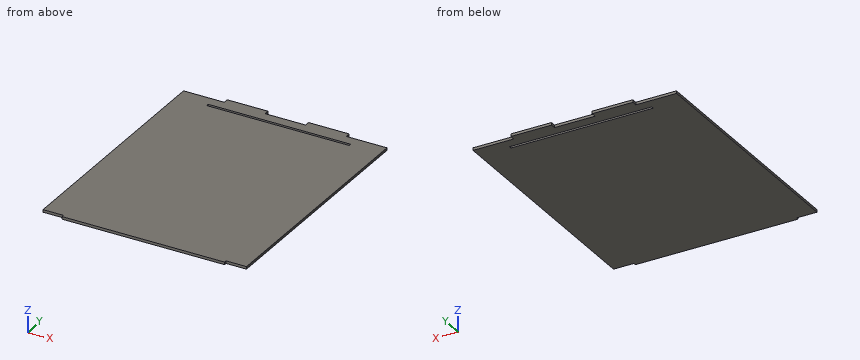
from build123d import *

# Parameters (mm, degrees)
SKETCH1_W           = 177.8
SKETCH1_H           = 3.175
BOSS_EXTRUDE1_DEPTH = 3.175


with BuildPart() as part:
    # Sketch1 → Boss-Extrude1 (new body)
    with BuildSketch(Plane.XY):
        Polygon((228.6, -6.35), (228.6, -3.175), (254, -3.175), (254, 301.625), (203.2, 301.625), (203.2, 307.975), (152.4, 307.975), (152.4, 301.625), (101.6, 301.625), (101.6, 307.975), (50.8, 307.975), (50.8, 301.625), (0, 301.625), (0, -3.175), (25.4, -3.175), (25.4, -6.35), align=None)
        with Locations((127, 287.3375)):
            Rectangle(SKETCH1_W, SKETCH1_H, mode=Mode.SUBTRACT)
    extrude(amount=BOSS_EXTRUDE1_DEPTH)


solid = part.part
Design review of the part built by this model. Coordinates are the model's own, in mm. Round coordinates to 2 decimals unless told otherwise and drop trailing zeros. Loops run counter-clockwise (first coordinate to the right, second up) from the corner with the lowest first, then second, coordinate; pieces in that order, holes last. Notation, with made-up numbers: (-6, 65.5) -> (21, 65.5) arc R15 ccw to (21, 90.5) -> close; hole circle Ø5 at (-35, -0.75). An arc over 180 degrees is marked (long way). Use one line per item in the form item = value. Start each with the question number.
Q1. We need section C-C on x = 225. Give the boundary of the cut face in (y, z) (3 decimals), then the cut area to 3 significant figures.
Q2. For pin 1 Ø1.6 at (y, z) = (303.5, 2) entering from -X; pin 2 Ø1.6 at (x, z) = (13.5, 1.5) entering from -Y (3 decimals), all flat-tipped, find the tip position at first contact; note any pin that passes through.
Q3. We need section B-B on z = 0.55. Give the boundary of the cut face in (x, y) (3 decimals), then the cut area to 3 significant figures.
Q4. Wall thickness on line 1 along Y through (x, z) = (51.5, 1.25) (3 decimals); line 2 along Y through (x, z) = (134, 2.7) (3 decimals); line 3 along Y through (x, z) = (11, 1.25) (3 decimals): over which ranges is each line inside the solid? List them lowest first. Write a range as [from, to].
Q5. We need section A-A on x = 108.5. Give the boundary of the cut face in (y, z) (3 decimals), then the cut area to 3 significant figures.
Calculated:
q1.outline = (-6.35, 0) -> (301.625, 0) -> (301.625, 3.175) -> (-6.35, 3.175) -> close
q1.area = 978 mm²
q2.pin_1 = 50.8
q2.pin_2 = -3.175
q3.outline = (0, -3.175) -> (25.4, -3.175) -> (25.4, -6.35) -> (228.6, -6.35) -> (228.6, -3.175) -> (254, -3.175) -> (254, 301.625) -> (203.2, 301.625) -> (203.2, 307.975) -> (152.4, 307.975) -> (152.4, 301.625) -> (101.6, 301.625) -> (101.6, 307.975) -> (50.8, 307.975) -> (50.8, 301.625) -> (0, 301.625) -> close; hole (38.1, 285.75) -> (215.9, 285.75) -> (215.9, 288.925) -> (38.1, 288.925) -> close
q3.area = 78,100 mm²
q4.line_1 = [-6.35, 285.75], [288.925, 307.975]
q4.line_2 = [-6.35, 285.75], [288.925, 301.625]
q4.line_3 = [-3.175, 301.625]
q5.outline = (-6.35, 0) -> (285.75, 0) -> (285.75, 3.175) -> (-6.35, 3.175) -> close; (288.925, 0) -> (301.625, 0) -> (301.625, 3.175) -> (288.925, 3.175) -> close
q5.area = 968 mm²
